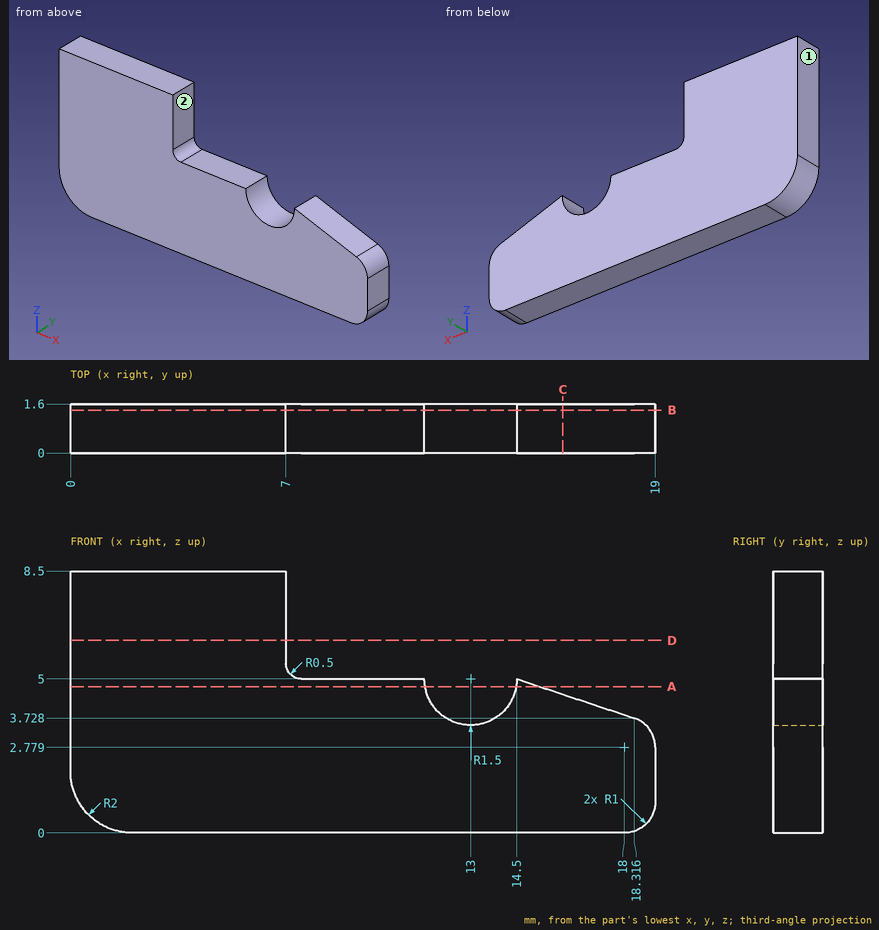
Design review of the part shown in the three views and the two pictorial views. Dimensions are in mm from the part's minimum x, y and z. A direction names the side the tool comes from. Give positions to 0.01 mm unless a question says otherwise; leave off trailing zeros. Order: outer loops, then holes, each group sorted by start corner. A loop starts at its lowest first (then second) coordinate and runs counter-clockwise, first axis right, second up. Notation, with made-up numbers: (20, 27) -> (54, 27) arc R22 ccw to (54, 57) -> close; hole circle Ø4 at (-3, -12.5). An arc over 180 degrees is marked (long way). Write each question's results on one line, items separated by ' | '. Start each with the question number.
Q1. Add section B-B on y = 1.4. Give the boundary of the cut face in (x, z).
Q2. Add section D-D on z = 6.25. Give the boundary of the cut face in (x, y), and give its area (3 significant figures).
Q3. For pin 1 (0.5 mm diameter, centred on x = 10, y = 0.5, fed in from +Z); pin 2 (0.8 mm diameter, centred on y = 0.5, z = 6.5, fed in from +X), all flat-tipped, find the tip position at first contact; note any pin that passes through.
Q4. Wall thickness on L1, parallel to Z at x = 9.5, y = 0.2; L2, parallel to X at y = 1.55, z = 7; L3, parallel to Z at x = 12.5, y = 1.2 (1 decimal): over which ranges is each line inside the solid? List them lowest first. Write a range as from..to.
Q5. Add section C-C on x = 16. Give the boundary of the cut face in (y, z).
Q6. Add section A-A on z = 4.75. Give the boundary of the cut face in (x, y).
Q7. Machinability: for the marked faces 1 and 2, which of the approach directions +Z, -Z, +X, -X, +Y, -Y give a long, thin tool a straight path to every point of the face, cutting with its end or side? Answer none if there is none.
Found:
1) outline: (0, 2) arc R2 ccw to (2, 0) -> (18, 0) arc R1 ccw to (19, 1) -> (19, 2.78) arc R1 ccw to (18.32, 3.73) -> (14.5, 5) arc R1.5 cw to (11.5, 5) -> (7.5, 5) arc R0.5 cw to (7, 5.5) -> (7, 8.5) -> (0, 8.5) -> close
2) outline: (0, 0) -> (7, 0) -> (7, 1.6) -> (0, 1.6) -> close | area: 11.2 mm2
3) pin 1: stops at z = 5 | pin 2: stops at x = 7
4) L1: z = 0..5 | L2: x = 0..7 | L3: z = 0..3.6
5) outline: (0, 0) -> (1.6, 0) -> (1.6, 4.5) -> (0, 4.5) -> close
6) outline: (0, 0) -> (11.52, 0) -> (11.52, 1.6) -> (0, 1.6) -> close; (14.48, 0) -> (15.25, 0) -> (15.25, 1.6) -> (14.48, 1.6) -> close
7) face 1: +Z, -Z, -X, +Y, -Y | face 2: +Z, +X, +Y, -Y
